from build123d import *

# Parameters (mm, degrees)
ESQUISSE1_R        = 4.25
BOSS_EXTRU_1_DEPTH = 2.5


with BuildPart() as part:
    # Esquisse1 → Boss.-Extru.1 (new body, symmetric)
    with BuildSketch(Plane.XY):
        Polygon((-4.618802154, -8), (4.618802154, -8), (9.237604307, 0), (4.618802154, 8), (-4.618802154, 8), (-9.237604307, 0), align=None)
        Circle(ESQUISSE1_R, mode=Mode.SUBTRACT)
    extrude(amount=BOSS_EXTRU_1_DEPTH, both=True)

    # Esquisse3 → Enlèvement de matière-Révolution2 (revolve, cut)
    with BuildSketch(Plane(origin=(0, 0, 0), x_dir=(0, 0, -1), z_dir=(1, 0, 0)), mode=Mode.PRIVATE) as enl_vement_de_mati_re_r_volution2_sk:
        with BuildLine():
            Line((3, 10.101429963), (3, 8))
            Line((3, 8), (2.5, 8))
            ThreePointArc((2.5, 8), (2.166714284, 9.000572077), (1.3, 9.601429963))
            Line((1.3, 9.601429963), (1.3, 10.101429963))
            Line((1.3, 10.101429963), (3, 10.101429963))
        make_face()
    enl_vement_de_mati_re_r_volution2 = revolve(enl_vement_de_mati_re_r_volution2_sk.sketch.rotate(Axis((0, 0, 5.617054836), (0, 0, -1)), 90), axis=Axis((0, 0, 5.617054836), (0, 0, -1)), mode=Mode.SUBTRACT)  # turned: the seam where the file's is

    # Symétrie1: Enlèvement de matière-Révolution2 across plane
    add(enl_vement_de_mati_re_r_volution2.mirror(Plane.XY), mode=Mode.SUBTRACT)


solid = part.part
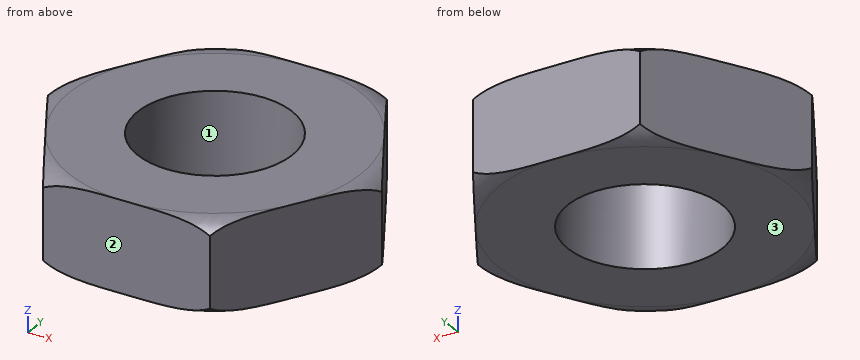
Read the model definition and answer for the solid it produces. Units are mm, in the model's axes. Face numbers are marked on the shaded views. Give positions to 0.01 mm unless a question says otherwise; leave off trailing zeros. Write each loop counter-clockwise with the first axis right and the second up, starting at its lowest first coordinate (ties: lowest second). Pieces come first, ordered by that corner, then holes. Notation, with made-up numbers: (64, -23) -> (83, -23) arc R8 ccw to (83, -14) -> close; hole circle Ø3 at (27, -1.75). An arc over 180 degrees is marked (long way). Answer as a JSON object with one key per item and string values. Group by question number.
1) Find section B-B (z = 2.2). Write down the section's boundary in (x, y), and give its area (3 significant figures).
2) Find section A-A (z = -0.05). Write down the section's boundary in (x, y).
3) Consider L1, parallel to X at y = -1, z = -0.6; L2, parallel to X at y = 3.25, z = 0.25; L3, parallel to Y at x = -2.25, z = 2. Determine where each line is inside the solid, lowest interval first. Write a range as from..to.
4) The mould has two halves that part along Y. Classify the marked faces 1, 2 and 3: +Y half, -Y half, draft (parallel to the pull), parting line (faces both ways), or undercut.
Values follow:
{
 "1": {"outline": "(-8.94, -0.52) -> (-4.92, -7.48) arc R8.95 ccw to (-4.02, -8) -> (4.02, -8) arc R8.95 ccw to (4.92, -7.48) -> (8.94, -0.52) arc R8.95 ccw to (8.94, 0.52) -> (4.92, 7.48) arc R8.95 ccw to (4.02, 8) -> (-4.02, 8) arc R8.95 ccw to (-4.92, 7.48) -> (-8.94, 0.52) arc R8.95 ccw to start; hole circle Ø8.5 at (0, 0)", "area": "164 mm2"},
 "2": {"outline": "(-9.24, 0) -> (-4.62, -8) -> (4.62, -8) -> (9.24, 0) -> (4.62, 8) -> (-4.62, 8) -> close; hole circle Ø8.5 at (0, 0)"},
 "3": {"L1": "x = -8.66..-4.13, 4.13..8.66", "L2": "x = -7.36..-2.74, 2.74..7.36", "L3": "y = -8..-3.61, 3.61..8"},
 "4": {"face 1": "undercut", "face 2": "-Y half", "face 3": "draft"}
}
